Here's how the part is built. I have some questions about the finished solid (model axes, mm). A direction names the side the tool comes from. Give positions to 0.01 mm unless a question says otherwise; leave off trailing zeros. Write each loop counter-clockwise with the first axis right and the second up, starting at its lowest first coordinate (ties: lowest second). Pieces come first, ordered by that corner, then holes. Notation, with made-up numbers: (-3, -12.75) -> (1, -12.75) arc R31 cw to (1, 18.25) -> close; hole circle Ø8 at (9, 50.5). An arc over 180 degrees is marked (long way). Answer as CSV lines item,"result". Start each with the question number.
Autodesk Inventor part; units mm, degrees
ref_plane "YZ Plane" through (0, 0, 0) normal (1, 0, 0) x (0, 1, 0)
ref_plane "XZ Plane" through (0, 0, 0) normal (0, 1, 0) x (-1, 0, 0)
ref_plane "XY Plane" through (0, 0, 0) normal (0, 0, 1) x (1, 0, 0)
sketch "Sketch1" plane through (0, 0, 0) normal (0, 0, 1) x (1, 0, 0)
  line L0 (-4.6523, 10.5287) -> (7.3477, 10.5287)
  line L1 (7.3477, 10.5287) -> (7.3477, -18.9713)
  line L2 (7.3477, -18.9713) -> (-4.6523, -18.9713)
  line L3 (-4.6523, -18.9713) -> (-4.6523, 10.5287)
  line L4 (-4.6523, 10.5287) -> (-4.6523, 16.5287)
  line L5 (-4.6523, 16.5287) -> (7.3477, 16.5287)
  line L6 (7.3477, 16.5287) -> (7.3477, 10.5287)
  line L7 (-4.6523, -18.9713) -> (-4.6523, -24.9713)
  line L8 (-4.6523, -24.9713) -> (7.3477, -24.9713)
  line L9 (7.3477, -24.9713) -> (7.3477, -18.9713)
  circle A0 centre (1.3477, 14.0287) radius 1.5
  circle A1 centre (1.3477, -22.4713) radius 1.5
  point P0 (0, 0)
  dimension "d0" = 12
  dimension "d1" = 29.5
  dimension "d2" = 6
  dimension "d3" = 6
  dimension "d4" = 3
  dimension "d5" = 3
  dimension "d23" = 2.5
  dimension "d24" = 2.5
  dimension "d25" = 3.5
  dimension "d26" = 6
  dimension "d27" = 6
extrude "Extrusion1" add sketch "Sketch1" against normal blind 20 contours L0 L1 L2 L3
extrude "Extrusion2" add sketch "Sketch1" against normal blind 2 contours L4 L5 L6 L0 | L2 L9 L8 L7
extrude "Extrusion3" add sketch "Sketch1" along normal blind 8 contours L0 L1 L2 L3
sketch "Sketch3" plane through (0, 0, 8) normal (0, 0, 1) x (1, 0, 0)
  line L0 (-4.6523, 10.5287) -> (7.3477, 10.5287)
  circle A0 centre (1.3477, 0.5287) radius 2.85
  line L1 (-4.6523, -18.9713) -> (-4.6523, 10.5287)
  point P0 (0, 0)
  dimension "d18" = 5.7
  dimension "d19" = 10
  dimension "d28" = 6
extrude "Extrusion5" add sketch "Sketch3" along normal blind 3.6
properties part number "GWS servo micro MG"
Item 1: If we section it at D-D (z = 5): Please give me the cut outline in (x, y), and give its area (3 significant figures).
Item 2: If we section it at B-B (x = 0.75): Please give me the cut outline in (y, z), and give its area (3 significant figures).
Item 3: If we section it at C-C (y = -4): Please give me the cut outline in (x, z), and give its area (3 significant figures).
Item 4: We'd pull the mould along Y, two halves only. Please class faces 4 (the face through (1, 10.529, -11)), 5 (the face through (1.023, 12.564, -0.986)), 6 (the face through (1, -24.971, -1)): released by +Y, released by -Y, zero draft, split by the parting line, or undercut.
Item 5: If I drill on line 1 (Z direction, x = 5, y = -10); line 2 (Y direction, x = -2.5, z = -10); line 3 (Z direction, x = -1, y = -23), over which ranges is the centre line in solid material (lowest first)? Write a range as [from, to].
Item 6: For faces 1 (the face through (1, 12, -2)), 2 (the face through (1.3, -20.6, -2)), 3 (the face through (1, -18.971, 4)), which set-ups out of +Z, -Z, +X, -X, +Y, -Y let a thin tool reach every point of the face, with its end or its side?
Item 7: I'm going to push flat-ended pins straight in: pin 1 (3.5 mm diameter, centred on x = 1.5, z = -15, fed in from +Y); pin 2 (3 mm diameter, centred on x = 0.5, y = 14, fed in from -Z); pin 3 (2 mm diameter, centred on x = -2, y = -10, fed in from +Z). Where does each tip first touch, or does it pass through?
Item 8: If we section it at A-A (x = 6): Please give me the cut outline in (y, z), and give its area (3 significant figures).
Final values:
1,outline,"(-4.65, -18.97) -> (7.35, -18.97) -> (7.35, 10.53) -> (-4.65, 10.53) -> close"
1,area,"354 mm2"
2,outline,"(-24.97, -2) -> (-23.85, -2) -> (-23.85, 0) -> (-24.97, 0) -> close; (-21.1, -2) -> (-18.97, -2) -> (-18.97, -20) -> (10.53, -20) -> (10.53, -2) -> (12.65, -2) -> (12.65, 0) -> (10.53, 0) -> (10.53, 8) -> (3.32, 8) -> (3.32, 11.6) -> (-2.26, 11.6) -> (-2.26, 8) -> (-18.97, 8) -> (-18.97, 0) -> (-21.1, 0) -> close; (15.4, -2) -> (16.53, -2) -> (16.53, 0) -> (15.4, 0) -> close"
2,area,"859 mm2"
3,outline,"(-4.65, -20) -> (7.35, -20) -> (7.35, 8) -> (-4.65, 8) -> close"
3,area,"336 mm2"
4,face 4,"released by +Y"
4,face 5,"undercut"
4,face 6,"released by -Y"
5,line 1,"[-20, 8]"
5,line 2,"[-18.97, 10.53]"
5,line 3,"[-2, 0]"
6,face 1,"-Z, +X, -X, +Y"
6,face 2,"-Z, +X, -X, -Y"
6,face 3,"+Z, +X, -X, -Y"
7,pin 1,"y = 10.53"
7,pin 2,"z = -2"
7,pin 3,"z = 8"
8,outline,"(-24.97, -2) -> (-18.97, -2) -> (-18.97, -20) -> (10.53, -20) -> (10.53, -2) -> (16.53, -2) -> (16.53, 0) -> (10.53, 0) -> (10.53, 8) -> (-18.97, 8) -> (-18.97, 0) -> (-24.97, 0) -> close"
8,area,"850 mm2"
